Part model, mm, in its own coordinate system. Face numbers are marked on the shaded views. A direction names the side the tool comes from. Coordinates: 2 decimals unless noted, no trailing zeros. Write each loop counter-clockwise with the first axis right and the second up, starting at its lowest first coordinate (ties: lowest second). Pieces come first, ordered by that corner, then holes. Notation, with made-up numbers: (-5, 82.25) - (45, 82.25) arc R27 ccw to (45, 119.25) - close; hole circle Ø11 at (77, 9.5). An arc over 180 degrees is marked (long way). Use a Markdown table: item, result.
```python
from build123d import *

# Parameters (mm, degrees)
F2_W      = 42
F2_H      = 42
F3_DEPTH  = 48
F4_R      = 1.5
F5_DEPTH  = 7
F4_R_2    = 11
F6_DEPTH  = 2
F7_R      = 2.5
F8_DEPTH  = 22
F10_DEPTH = 17
F11_SIZE  = 3
F12_R     = 0.5
F13_R     = 0.5
F14_R     = 0.5


with BuildPart() as f3:
    # F2 (on Top) → F3 (new body)
    with BuildSketch(Plane.XY):
        Rectangle(F2_W, F2_H)
    extrude(amount=F3_DEPTH)

    # F4 (on face) → F5 (cut)
    with BuildSketch(Plane.XY.offset(48)):
        with Locations((-15.5, -15.5)):
            Circle(F4_R)
        with Locations((-15.5, 15.5)):
            Circle(F4_R)
        with Locations((15.5, 15.5)):
            Circle(F4_R)
        with Locations((15.5, -15.5)):
            Circle(F4_R)
    extrude(amount=-F5_DEPTH, mode=Mode.SUBTRACT)

    # F4 (on face) → F6 (join)
    with BuildSketch(Plane.XY.offset(48)):
        Circle(F4_R_2)
    extrude(amount=F6_DEPTH)

    # F7 (on face) → F8 (join)
    with BuildSketch(Plane.XY.offset(50)):
        Circle(F7_R)
    extrude(amount=F8_DEPTH)

    # F9 (on face) → F10 (cut)
    with BuildSketch(Plane.XY.offset(72)):
        with BuildLine():
            ThreePointArc((1.5, 2), (0, 2.5), (-1.5, 2))
            Line((-1.5, 2), (1.5, 2))
        make_face()
    extrude(amount=-F10_DEPTH, mode=Mode.SUBTRACT)

    # F11
    f11_edges = [f3.edges().sort_by_distance(p)[0] for p in [
        (21, -21, 24),
        (21, 21, 24),
        (-21, -21, 24),
        (-21, 21, 24),
    ]]
    chamfer(f11_edges, length=F11_SIZE)

    # F12
    f12_edges = [f3.edges().sort_by_distance(p)[0] for p in [
        (0, 21, 48),
        (19.5, 19.5, 48),
        (21, 0, 48),
        (19.5, -19.5, 48),
        (0, -21, 48),
        (-19.5, -19.5, 48),
        (-21, 0, 48),
        (-19.5, 19.5, 48),
    ]]
    fillet(f12_edges, radius=F12_R)

    # F13
    f13_edges = [f3.edges().sort_by_distance(p)[0] for p in [
        (-19.5, 19.5, 0),
        (0, 21, 0),
        (19.5, 19.5, 0),
        (21, 0, 0),
        (19.5, -19.5, 0),
        (0, -21, 0),
        (-19.5, -19.5, 0),
        (-21, 0, 0),
    ]]
    fillet(f13_edges, radius=F13_R)

    # F14
    f14_edges = [f3.edges().sort_by_distance(p)[0] for p in [
        (-11, 0, 50),
    ]]
    fillet(f14_edges, radius=F14_R)


solid = f3.part
```
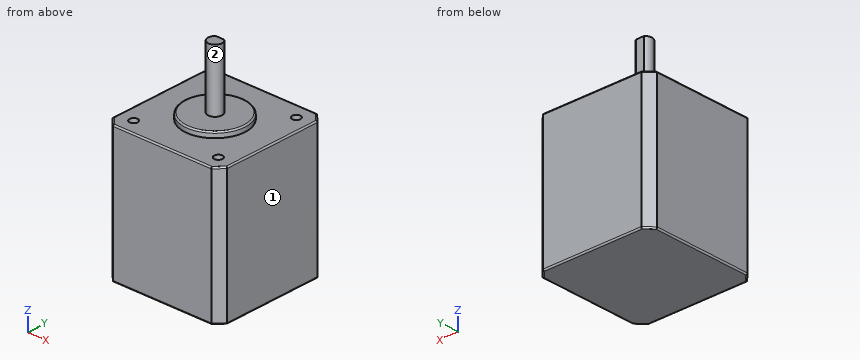
Item 1: Band-saw the part on C-C, the plane x = 0. Give the cut face in (y, z), then the cut area to 3 significant figures.
From the geometry:
| item | result |
|---|---|
| outline | (-21, 0.5) arc R0.5 ccw to (-20.5, 0) - (20.5, 0) arc R0.5 ccw to (21, 0.5) - (21, 47.5) arc R0.5 ccw to (20.5, 48) - (11, 48) - (11, 49.5) arc R0.5 ccw to (10.5, 50) - (2.5, 50) - (2.5, 55) - (2, 55) - (2, 72) - (-2.5, 72) - (-2.5, 50) - (-10.5, 50) arc R0.5 ccw to (-11, 49.5) - (-11, 48) - (-20.5, 48) arc R0.5 ccw to (-21, 47.5) - close |
| area | 2,160 mm^2 |
Item 2: Band-saw the part on B-B, the plane y = 12. Give the cut face in (x, z), then the cut area to 3 significant figures.
From the geometry:
| item | result |
|---|---|
| outline | (-21, 0.5) arc R0.5 ccw to (-20.5, 0) - (20.5, 0) arc R0.5 ccw to (21, 0.5) - (21, 47.5) arc R0.5 ccw to (20.5, 48) - (-20.5, 48) arc R0.5 ccw to (-21, 47.5) - close |
| area | 2,020 mm^2 |
Item 3: Drill centre lines: probe 1 along Y at (x, z) = (-15.5, 45); probe 2 along Y at (x, z) = (-15, 44). Where is each one in solid material? Low to high.
From the geometry:
| item | result |
|---|---|
| probe 1 | -21 to -17, -14 to 14, 17 to 21 |
| probe 2 | -21 to -16.91, -14.09 to 14.09, 16.91 to 21 |
Item 4: Which spindle directions (+Z, -Z, +X, -X, +Y, -Y) get a long thin tool onto all of the face, cutting with end or side? Do the marked faces 1 and 2. Say none if no direction does.
From the geometry:
| item | result |
|---|---|
| face 1 | +Z, -Z, +X, +Y, -Y |
| face 2 | +Z |
Item 5: Band-saw the part on D-D, the plane z = 51. Give the cut face in (x, y), then the cut area to 3 significant figures.
From the geometry:
| item | result |
|---|---|
| outline | circle Ø5 at (0, 0) |
| area | 19.6 mm^2 |
Item 6: Band-saw the part on A-A, the plane x = -15.5. Give the cut face in (y, z).
From the geometry:
| item | result |
|---|---|
| outline | (-21, 0.5) arc R0.5 ccw to (-20.5, 0) - (20.5, 0) arc R0.5 ccw to (21, 0.5) - (21, 47.5) arc R0.5 ccw to (20.5, 48) - (17, 48) - (17, 41) - (14, 41) - (14, 48) - (-14, 48) - (-14, 41) - (-17, 41) - (-17, 48) - (-20.5, 48) arc R0.5 ccw to (-21, 47.5) - close |
Item 7: Drop flat-ended pins along their axis: P1, Ø1.5, axis at x = -15, y = -15.5, coming from the +Z side; P2, Ø1, axis at x = 2.5, y = 11, coming from the +Z side; P3, Ø0.9, axis at x = -0.5, z = 59.5, coming from the +Y side; P4, Ø10.5, axis at x = -2.5, y = 3, coming from the +Z side. Give the stop position or say it passes through.
From the geometry:
| item | result |
|---|---|
| P1 | z = 41 |
| P2 | z = 49.91 |
| P3 | y = 2 |
| P4 | z = 72 |
